Here's how the part is built. I have some questions about the finished solid (model axes, mm). Face numbers are marked on the shaded views. Give positions to 0.01 mm unless a question says otherwise; leave off trailing zeros. Loops run counter-clockwise (first coordinate to the right, second up) from the corner with the lowest first, then second, coordinate; pieces in that order, holes last. Notation, with made-up numbers: (-3.75, 0.5) - (18.25, 0.5) arc R32 cw to (18.25, 39.5) - close; hole circle Ø9 at (-29, 44). An arc over 180 degrees is marked (long way). Use a Markdown table: item, result.
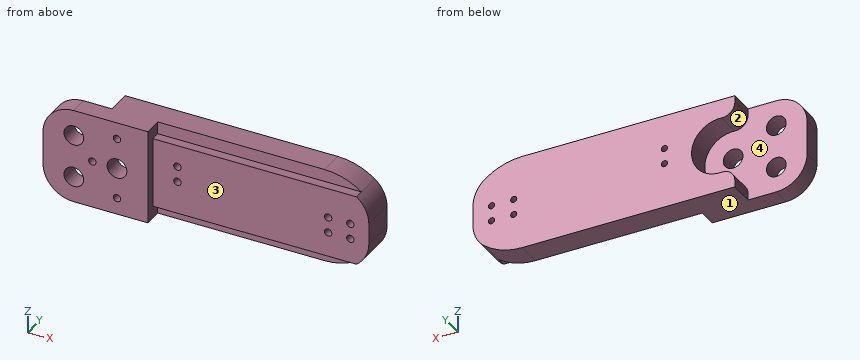
from build123d import *

# Parameters (mm, degrees)
SKETCH_2_W          = 35.05
SKETCH_2_H          = 11.3952
SKETCH_2_R          = 0.6
EXTRUDE_1_DEPTH     = 1.5
SKETCH_3_W          = 39.05
SKETCH_3_H          = 15.3952
SKETCH_3_R          = 0.5
EXTRUDE_2_DEPTH     = 4
SKETCH_4_W          = 15
SKETCH_4_H          = 4
EXTRUDE_3_DEPTH     = 15.3952
SKETCH_5_W          = 17
SKETCH_5_H          = 15.3952
EXTRUDE_4_DEPTH     = 3
SKETCH_6_R          = 1.6
CUT_EXTRUDE_1_DEPTH = 157.48252797
CUT_EXTRUDE_2_DEPTH = 4
CUT_EXTRUDE_4_DEPTH = 4
FILLET_2_R          = 5
CUT_EXTRUDE_5_DEPTH = 4
FILLET_3_R          = 2
SKETCH_10_R         = 0.6
CUT_EXTRUDE_6_DEPTH = 2
CUT_EXTRUDE_7_DEPTH = 157.422605654
CUT_EXTRUDE_8_DEPTH = 156.918332452
FILLET_5_R          = 5


with BuildPart() as part:
    # 草图2 → 凸台-拉伸1 (new body)
    with BuildSketch(Plane(origin=(0, 0, 0), x_dir=(1, 0, 0), z_dir=(0, 1, 0))):
        with Locations((108.28655231, 82.313447411)):
            Rectangle(SKETCH_2_W, SKETCH_2_H)
        with Locations(Location((94.76155231, 82.701047411, 0), (0, 0, 270))):
            Circle(SKETCH_2_R, mode=Mode.SUBTRACT)
        with Locations(Location((94.76155231, 80.161047411, 0), (0, 0, 270))):
            Circle(SKETCH_2_R, mode=Mode.SUBTRACT)
        with Locations(Location((119.21155231, 84.011047411, 0), (0, 0, 270))):
            Circle(SKETCH_2_R, mode=Mode.SUBTRACT)
        with Locations(Location((122.81155231, 84.011047411, 0), (0, 0, 270))):
            Circle(SKETCH_2_R, mode=Mode.SUBTRACT)
        with Locations(Location((122.81155231, 81.471047411, 0), (0, 0, 270))):
            Circle(SKETCH_2_R, mode=Mode.SUBTRACT)
        with Locations(Location((119.21155231, 81.471047411, 0), (0, 0, 270))):
            Circle(SKETCH_2_R, mode=Mode.SUBTRACT)
    extrude(amount=EXTRUDE_1_DEPTH)

    # 草图3 → 凸台-拉伸2 (add)
    with BuildSketch(Plane(origin=(0, 1.5, 0), x_dir=(1, 0, 0), z_dir=(0, 1, 0))):
        with Locations((108.28655231, 82.313447411)):
            Rectangle(SKETCH_3_W, SKETCH_3_H)
        with Locations(Location((94.76155231, 82.701047411, 0), (0, 0, 270))):
            Circle(SKETCH_3_R, mode=Mode.SUBTRACT)
        with Locations(Location((94.76155231, 80.161047411, 0), (0, 0, 270))):
            Circle(SKETCH_3_R, mode=Mode.SUBTRACT)
        with Locations(Location((119.21155231, 84.011047411, 0), (0, 0, 270))):
            Circle(SKETCH_3_R, mode=Mode.SUBTRACT)
        with Locations(Location((122.81155231, 84.011047411, 0), (0, 0, 270))):
            Circle(SKETCH_3_R, mode=Mode.SUBTRACT)
        with Locations(Location((122.81155231, 81.471047411, 0), (0, 0, 270))):
            Circle(SKETCH_3_R, mode=Mode.SUBTRACT)
        with Locations(Location((119.21155231, 81.471047411, 0), (0, 0, 270))):
            Circle(SKETCH_3_R, mode=Mode.SUBTRACT)
    extrude(amount=EXTRUDE_2_DEPTH)

    # 草图4 → 凸台-拉伸3 (add)
    with BuildSketch(Plane(origin=(0, 0, -90.011047411), x_dir=(-1, 0, 0), z_dir=(0, 0, -1))):
        with Locations((-81.26155231, 3.5)):
            Rectangle(SKETCH_4_W, SKETCH_4_H)
    extrude(amount=-EXTRUDE_3_DEPTH)

    # 草图5 → 凸台-拉伸4 (add)
    with BuildSketch(Plane.XZ.offset(-1.5)):
        with Locations((82.26155231, -82.313447411)):
            Rectangle(SKETCH_5_W, SKETCH_5_H)
    extrude(amount=EXTRUDE_4_DEPTH)

    # 草图6 → 切除-拉伸1 (cut, through all)
    with BuildSketch(Plane.XZ.offset(1.5)):
        with Locations(Location((78.76155231, -78.813447411, 0), (0, 0, 270))):
            Circle(SKETCH_6_R)
        with Locations(Location((85.76155231, -82.313447411, 0), (0, 0, 270))):
            Circle(SKETCH_6_R)
        with Locations(Location((78.76155231, -85.813447411, 0), (0, 0, 270))):
            Circle(SKETCH_6_R)
    extrude(amount=-CUT_EXTRUDE_1_DEPTH, mode=Mode.SUBTRACT)

    # 草图7 → 切除-拉伸2 (cut)
    with BuildSketch(Plane(origin=(0, 5.5, 0), x_dir=(1, 0, 0), z_dir=(0, 1, 0))):
        with BuildLine():
            ThreePointArc((83.342986542, 86.226315876), (76.648541293, 89.899421523), (75.776589998, 82.313447411))
            ThreePointArc((75.776589998, 82.313447411), (76.648541293, 74.727473299), (83.342986542, 78.400578945))
            ThreePointArc((83.342986542, 78.400578945), (90.36155231, 82.313447411), (83.342986542, 86.226315876))
        make_face()
    extrude(amount=-CUT_EXTRUDE_2_DEPTH, mode=Mode.SUBTRACT)

    # 草图8 → 切除-拉伸4 (cut)
    with BuildSketch(Plane(origin=(0, 5.5, 0), x_dir=(1, 0, 0), z_dir=(0, 1, 0))):
        with BuildLine():
            Line((76.880022549, 90.011047411), (73.76155231, 90.011047411))
            Line((73.76155231, 90.011047411), (73.76155231, 74.615847411))
            Line((73.76155231, 74.615847411), (76.880022549, 74.615847411))
            ThreePointArc((76.880022549, 74.615847411), (74.208097828, 78.160720601), (75.776589998, 82.313447411))
            ThreePointArc((75.776589998, 82.313447411), (74.208097828, 86.466174221), (76.880022549, 90.011047411))
        make_face()
    extrude(amount=-CUT_EXTRUDE_4_DEPTH, mode=Mode.SUBTRACT)

    # 圆角2
    fillet_2_edges = [part.edges().sort_by_distance(p)[0] for p in [
        (73.76155231, 0, -74.615847411),
        (73.76155231, 0, -90.011047411),
    ]]
    fillet(fillet_2_edges, radius=FILLET_2_R)

    # 草图9 → 切除-拉伸5 (cut)
    with BuildSketch(Plane(origin=(0, 5.5, 0), x_dir=(1, 0, 0), z_dir=(0, 1, 0))):
        Polygon((83.342986542, 86.226315876), (83.342986542, 90.011047411), (80.64308207, 90.011047411), align=None)
        Polygon((83.342986542, 78.400578945), (83.342986542, 74.615847411), (80.64308207, 74.615847411), align=None)
    extrude(amount=-CUT_EXTRUDE_5_DEPTH, mode=Mode.SUBTRACT)

    # 圆角3
    fillet_3_edges = [part.edges().sort_by_distance(p)[0] for p in [
        (83.342986542, 3.5, -78.400578945),
        (83.342986542, 3.5, -86.226315876),
    ]]
    fillet(fillet_3_edges, radius=FILLET_3_R)

    # 草图10 → 切除-拉伸6 (cut)
    with BuildSketch(Plane.XZ.offset(1.5)):
        with Locations(Location((81.76155231, -82.313447411, 0), (0, 0, 270))):
            Circle(SKETCH_10_R)
        with Locations(Location((85.76155231, -77.313447411, 0), (0, 0, 270))):
            Circle(SKETCH_10_R)
        with Locations(Location((85.76155231, -87.313447411, 0), (0, 0, 270))):
            Circle(SKETCH_10_R)
    extrude(amount=-CUT_EXTRUDE_6_DEPTH, mode=Mode.SUBTRACT)

    # 草图11 → 切除-拉伸7 (cut, through all)
    with BuildSketch(Plane.XZ):
        with BuildLine():
            Line((127.81155231, -74.615847411), (117.81155231, -74.615847411))
            ThreePointArc((117.81155231, -74.615847411), (120.97382997, -75.12901443), (123.811552309, -76.615847411))
            Line((123.811552309, -76.615847411), (125.81155231, -76.615847411))
            Line((125.81155231, -76.615847411), (125.81155231, -78.615847411))
            ThreePointArc((125.811552309, -78.615847411), (126.278688967, -79.295359009), (126.688253102, -80.011047411))
            ThreePointArc((126.688253102, -80.011047411), (127.249902706, -82.313447411), (126.688253102, -84.615847411))
            ThreePointArc((126.688253102, -84.615847411), (126.278688967, -85.331535812), (125.811552309, -86.011047411))
            Line((125.81155231, -86.011047411), (125.81155231, -88.011047411))
            Line((125.81155231, -88.011047411), (123.811552309, -88.011047411))
            ThreePointArc((123.811552309, -88.011047411), (120.97382997, -89.497880391), (117.81155231, -90.011047411))
            Line((117.81155231, -90.011047411), (127.81155231, -90.011047411))
            Line((127.81155231, -90.011047411), (127.811552309, -84.615847411))
            Line((127.811552309, -84.615847411), (127.811552309, -80.011047411))
            Line((127.811552309, -80.011047411), (127.81155231, -74.615847411))
        make_face()
        with BuildLine():
            Line((125.81155231, -76.615847411), (123.811552309, -76.615847411))
            ThreePointArc((123.811552309, -76.615847411), (124.882620121, -77.544779599), (125.811552309, -78.615847411))
            Line((125.81155231, -78.615847411), (125.81155231, -76.615847411))
        make_face()
        with BuildLine():
            Line((125.81155231, -88.011047411), (125.81155231, -86.011047411))
            ThreePointArc((125.811552309, -86.011047411), (124.882620121, -87.082115223), (123.811552309, -88.011047411))
            Line((123.811552309, -88.011047411), (125.81155231, -88.011047411))
        make_face()
    extrude(amount=-CUT_EXTRUDE_7_DEPTH, mode=Mode.SUBTRACT)

    # 草图12 → 切除-拉伸8 (cut, through all)
    with BuildSketch(Plane.XZ.offset(-1.5)):
        with BuildLine():
            Line((125.81155231, -78.615847411), (125.81155231, -86.011047411))
            ThreePointArc((125.81155231, -86.011047411), (126.278688967, -85.331535812), (126.688253102, -84.615847411))
            ThreePointArc((126.688253102, -84.615847411), (127.249902706, -82.313447411), (126.688253102, -80.011047411))
            ThreePointArc((126.688253102, -80.011047411), (126.278688967, -79.295359009), (125.81155231, -78.615847411))
        make_face()
    extrude(amount=-CUT_EXTRUDE_8_DEPTH, mode=Mode.SUBTRACT)

    # 圆角5
    fillet_5_edges = [part.edges().sort_by_distance(p)[0] for p in [
        (125.811552309, 2.75, -86.011047411),
        (125.811552309, 2.75, -78.615847411),
    ]]
    fillet(fillet_5_edges, radius=FILLET_5_R - 0.0001)  # a hair under: the kernel refuses the full size


solid = part.part
(1) Suppose I cut it at A-A on x = 104. Write out the boundary of the cut face in (y, z).
A:
| item | result |
|---|---|
| outline | (0, -88.01) - (1.5, -88.01) - (1.5, -90.01) - (5.5, -90.01) - (5.5, -74.62) - (1.5, -74.62) - (1.5, -76.62) - (0, -76.62) - close |
(2) Suppose I cut it at B-B on y = 1. Count the separate pieces of the cut face and the enclosed holes in it, plus the area to 3 significant figures.
A:
| item | result |
|---|---|
| separate pieces | 1 |
| enclosed holes | 9 |
| area | 615 mm2 |
(3) Will these pins go through, and if not, where does the flat tip stop? pin 1 (6 mm diameter, centred on x = 96.5, z = -83, fed in from -Y); pin 2 (1 mm diameter, centred on x = 109.5, z = -89, fed in from -Y); pin 3 (1.9 mm diameter, centred on x = 81.76, z = -82.31, fed in from +Y).
A:
| item | result |
|---|---|
| pin 1 | y = 0 |
| pin 2 | y = 1.5 |
| pin 3 | y = 1.5 |
(4) If I drill on line 1 (Y direction, x = 79, z = -82.25); line 2 (Y direction, x = 109.5, z = -88.25); line 3 (X direction, y = 1.25, z = -86.75), over which ranges is the centre line in solid material (lowest first)?
A:
| item | result |
|---|---|
| line 1 | -1.5 to 1.5 |
| line 2 | 1.5 to 5.5 |
| line 3 | 74.07 to 77.46, 80.06 to 124.99 |
(5) Suppose I cut it at C-C on x = 121.5. Write out the boundary of the cut face in (y, z).
A:
| item | result |
|---|---|
| outline | (0, -88.01) - (1.5, -88.01) - (1.5, -89.31) - (5.5, -89.31) - (5.5, -75.32) - (1.5, -75.32) - (1.5, -76.62) - (0, -76.62) - close |
(6) We'd pull the mould along Z, two halves only. Please class the marked faces 1, 2, 3 and 4: pulls with the +Z half, pulls with the -Z half, needs draft (parallel to the pull), parting line crosses it, or undercut.
A:
| item | result |
|---|---|
| face 1 | pulls with the -Z half |
| face 2 | undercut |
| face 3 | needs draft |
| face 4 | undercut |
